Autodesk Inventor part; units mm, degrees
ref_plane "YZ Plane" through (0, 0, 0) normal (1, 0, 0) x (0, 1, 0)
ref_plane "XZ Plane" through (0, 0, 0) normal (0, 1, 0) x (-1, 0, 0)
ref_plane "XY Plane" through (0, 0, 0) normal (0, 0, 1) x (1, 0, 0)
sketch "Sketch1" plane through (0, 0, 0) normal (0, 0, 1) x (1, 0, 0)
  line L0 (50, -50) -> (-50, -50)
  line L1 (-50, -50) -> (-50, 50)
  line L2 (-50, 50) -> (50, 50)
  line L3 (50, 50) -> (50, -50)
  line L4 (50, -50) -> (-50, 50) construction
  line L5 (-50, -50) -> (50, 50) construction
  point P0 (0, 0)
  dimension "d0" = 100
extrude "Extrusion1" add sketch "Sketch1" along normal blind 3
sketch "Sketch2" plane through (0, 0, 3) normal (0, 0, 1) x (1, 0, 0)
  line L0 (-50, 50) -> (-50, -50) construction
  line L1 (-47, 40) -> (-50, 40)
  line L2 (-50, 40) -> (-50, 50)
  line L3 (-50, 50) -> (-47, 50)
  line L4 (-47, 50) -> (-47, 40)
  line L5 (-47, 40) -> (-50, 50) construction
  line L6 (-50, 40) -> (-47, 50) construction
  point P0 (0, 0)
  point P1 (-48.5, 45)
  dimension "d3" = 10
  dimension "d4" = 3
extrude "Extrusion2" cut sketch "Sketch2" against normal through all
pattern_linear "Rectangular Pattern1" count 5 spacing 20 along (0, -1, 0) of "Extrusion2"
pattern_circular "Circular Pattern1" count 4 over 360 about axis through (0, 0, -10) along (0, 0, 1) of "Extrusion2", "Rectangular Pattern1"
sketch "Sketch3" plane through (0, 0, 3) normal (0, 0, 1) x (1, 0, 0)
  line L0 (15.5, -15.5) -> (-15.5, -15.5) construction
  line L1 (-15.5, -15.5) -> (-15.5, 15.5) construction
  line L2 (-15.5, 15.5) -> (15.5, 15.5) construction
  line L3 (15.5, 15.5) -> (15.5, -15.5) construction
  line L4 (15.5, -15.5) -> (-15.5, 15.5) construction
  line L5 (-15.5, -15.5) -> (15.5, 15.5) construction
  circle A0 centre (-15.5, 15.5) radius 1.6
  circle A1 centre (-15.5, -15.5) radius 1.6
  circle A2 centre (15.5, -15.5) radius 1.6
  circle A3 centre (15.5, 15.5) radius 1.6
  circle A4 centre (0, 0) radius 11.5
  dimension "d13" = 31
  dimension "d14" = 3.2
  dimension "d17" = 23
extrude "Extrusion3" cut sketch "Sketch3" against normal through all
properties part number "Base"
Input: part model. Units: mm. Frame: model coordinates. A direction names the side the tool comes from. Round coordinates to 2 decimals unless told otherwise and drop trailing zeros. Order: outer loops, then holes, each group sorted by start corner. A loop starts at its lowest first (then second) coordinate and runs counter-clockwise, first axis right, second up.
1. Cut plane C-C, the plane x = -5. Output: boundary loops of the cut face in (y, z).
The answers:
outline: (-47, 0) - (-10.36, 0) - (-10.36, 3) - (-47, 3) - close; (10.36, 0) - (50, 0) - (50, 3) - (10.36, 3) - close
2. Material intervals for line 1 (Y direction, x = 15.5, z = 1.3); line 2 (Y direction, x = -15.5, z = 2.4); line 3 (X direction, y = 24, z = 0.85), sorted ascending.
The answers:
line 1: y = -47 to -17.1, -13.9 to 13.9, 17.1 to 50
line 2: y = -50 to -17.1, -13.9 to 13.9, 17.1 to 47
line 3: x = -47 to 50
3. Mould query, pull axis X, two halves, no side actions, for faces 1 (the face through (-48, 0, 2)), 2 (the face through (-50, -25, 1)), 3 (the face through (40, -48, 2)). Classes: released by +X, released by -X, zero draft, split by the parting line, or undercut.
The answers:
face 1: zero draft
face 2: released by -X
face 3: undercut
4. Cut plane D-D, the plane z = 0.8. State how many separate pieces and enclosed holes the cut face has, then the cut area to 3 significant figures.
The answers:
separate pieces: 1
enclosed holes: 5
area: 8,950 mm2
5. Pin query (flat end, axial travel): P1, Ø1.5, axis at x = -48.5, z = 1.5, coming from the -Y side; P2, Ø1.5, axis at y = -48, z = 1.5, coming from the -X side; P3, Ø1.5, axis at y = -24.5, z = 2, coming from the +X side. Return the tip coordinate at first contact, or that it passes through.
The answers:
P1: stops at y = -47
P2: stops at x = -40
P3: stops at x = 47
6. Set-up query: faces 4 (the face through (50, 44, 1)), 5 (the face through (47, -45, 2)), 6 (the face through (-30, 49, 2)), 7 (the face through (-47, 5, 2)), 8 (the face through (48, -20, 2)). Return all of +Z, -Z, +X, -X, +Y, -Y with unobstructed straight access to the full face (end or side cutting, diameter ignored); none if empty.
The answers:
face 4: +Z, -Z, +X, +Y, -Y
face 5: +Z, -Z, +X, -Y
face 6: +Z, -Z, +Y
face 7: +Z, -Z, -X
face 8: +Z, -Z, +X
7. Cut plane A-A, the plane x = 15.5. Output: boundary loops of the cut face in (y, z), then the cut area to 3 significant figures.
The answers:
outline: (-47, 0) - (-17.1, 0) - (-17.1, 3) - (-47, 3) - close; (-13.9, 0) - (13.9, 0) - (13.9, 3) - (-13.9, 3) - close; (17.1, 0) - (50, 0) - (50, 3) - (17.1, 3) - close
area: 272 mm2
8. Cut plane B-B, the plane y = 15.5. Output: boundary loops of the cut face in (x, z), then the cut area to 3 significant figures.
The answers:
outline: (-50, 0) - (-17.1, 0) - (-17.1, 3) - (-50, 3) - close; (-13.9, 0) - (13.9, 0) - (13.9, 3) - (-13.9, 3) - close; (17.1, 0) - (47, 0) - (47, 3) - (17.1, 3) - close
area: 272 mm2
